Source: three-view drawing plus pictorial views. Frame: mm from the lowest corner of the part. A direction names the side the tool comes from. Give positions to 0.01 mm unless a question says otherwise; leave off trailing zeros. Write each loop counter-clockwise with the first axis right and the second up, starting at its lowest first coordinate (ties: lowest second). Pieces come first, ordered by that corner, then holes.
Q1. Cut plane B-B on z = 10.5. Return the cut outline in (x, y) (3 decimals).
Q2. Cut plane C-C on y = 3.25. Return the cut outline in (x, z), plus the area to 3 significant figures.
Q3. Cut plane A-A on x = 12.5. Return the cut outline in (y, z) (3 decimals), plus the area to 3 significant figures.
Q4. Draft query along Z for the marked faces 3, 4 and 5. Return one class per face: pulls with the +Z half, pulls with the -Z half, needs draft (parallel to the pull), parting line crosses it, or undercut.
Q5. Pin query (flat end, axial travel): pin 1 (3 mm diameter, centred on x = 15, z = 10.5, fed in from -Y) (3 decimals); pin 2 (1.5 mm diameter, centred on x = 4.5, y = 3.5, fed in from +Z); pin 3 (1 mm diameter, centred on x = 12, z = 14, fed in from +Y) (3 decimals). Return the tip coordinate at first contact, or that it passes through.
Q6. Line query: L1, parallel to Z at x = 12.5, y = 0.6; L2, parallel to Y at x = 20.5, z = 8.5 (3 decimals). Output: solid intervals per line, ascending.
Q7. Reachability of the marked faces 1 and 2 from +Z, -Z, +X, -X, +Y, -Y: full face, straight path, thin tool, end or side. Return the list, or none.
Q8. Cut plane D-D on x = 23.5. Return the cut outline in (y, z).
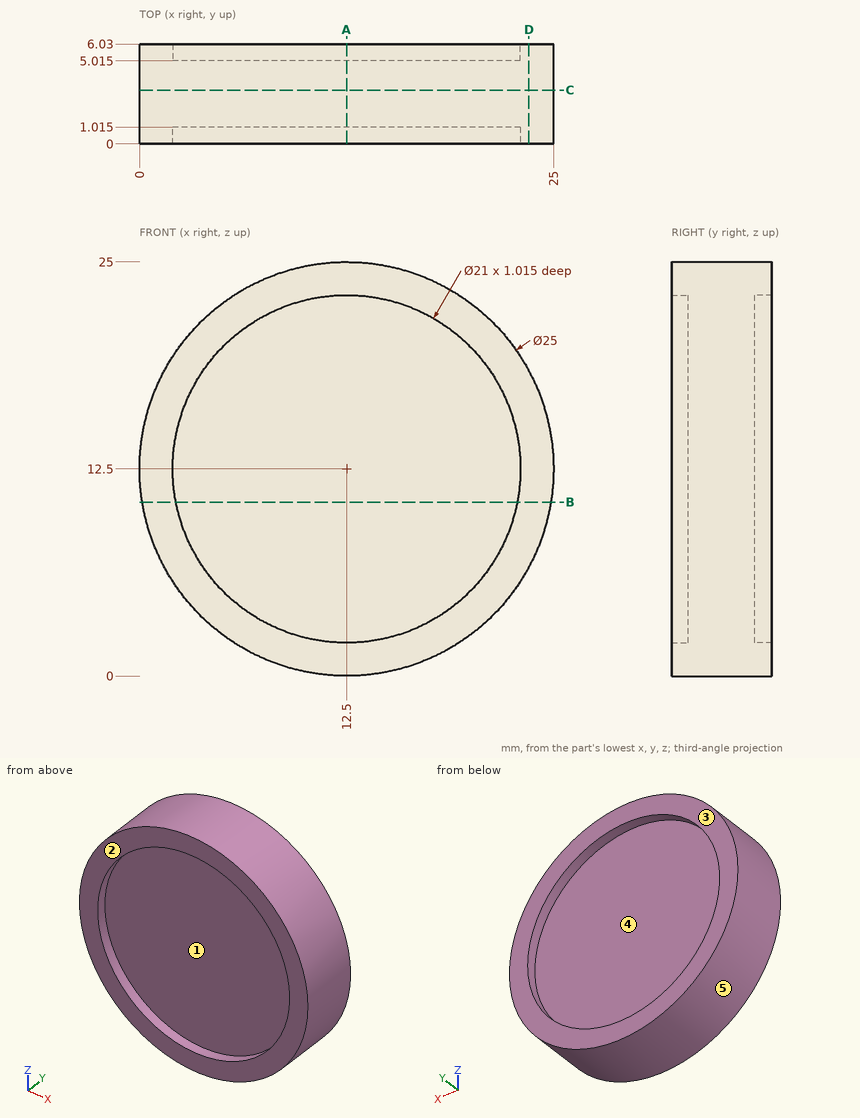
Data:
1. outline: (0.161, 0) - (2.192, 0) - (2.192, 1.015) - (22.808, 1.015) - (22.808, 0) - (24.839, 0) - (24.839, 6.03) - (22.808, 6.03) - (22.808, 5.015) - (2.192, 5.015) - (2.192, 6.03) - (0.161, 6.03) - close
2. outline: circle Ø25 at (12.5, 12.5)
2. area: 491 mm2
3. outline: (0, 0) - (6.03, 0) - (6.03, 2) - (5.015, 2) - (5.015, 23) - (6.03, 23) - (6.03, 25) - (0, 25) - (0, 23) - (1.015, 23) - (1.015, 2) - (0, 2) - close
3. area: 108 mm2
4. face 3: needs draft
4. face 4: undercut
4. face 5: parting line crosses it
5. pin 1: stops at y = 1.015
5. pin 2: stops at z = 22.68
5. pin 3: stops at y = 5.015
6. L1: z = 0 to 2, 23 to 25
6. L2: y = 1.015 to 5.015
7. face 1: -Y
7. face 2: +Z, -Z, +X, -X, -Y
8. outline: (0, 6.56) - (6.03, 6.56) - (6.03, 18.44) - (0, 18.44) - close
